from build123d import *

# Parameters (mm, degrees)
SKETCH1_R      = 3.96875
EXTRUDE1_DEPTH = 31.75
CHAMFER1_SIZE  = 0.7874
SKETCH2_W      = 7.62
SKETCH2_H      = 1.27
EXTRUDE2_DEPTH = 6.35


with BuildPart() as part:
    # Sketch1 → Extrude1 (new body)
    with BuildSketch(Plane(origin=(0, 0, 0), x_dir=(0, 0, -1), z_dir=(1, 0, 0))):
        Circle(SKETCH1_R)
    extrude(amount=EXTRUDE1_DEPTH)

    # Chamfer1
    chamfer1_edges = [part.edges().sort_by_distance(p)[0] for p in [
        (0, 0, 3.96875),
        (31.75, 0, 3.96875),
    ]]
    chamfer(chamfer1_edges, length=CHAMFER1_SIZE)

    # Sketch2 → Extrude2 (cut)
    with BuildSketch(Plane(origin=(31.75, 0, 0), x_dir=(0, 0, -1), z_dir=(1, 0, 0))):
        with Locations((0, 3.82905)):
            Rectangle(SKETCH2_W, SKETCH2_H)
    extrude(amount=-EXTRUDE2_DEPTH, mode=Mode.SUBTRACT)


solid = part.part
Read the model definition and answer for the solid it produces. Units are mm, in the model's axes. A direction names the side the tool comes from. Round coordinates to 2 decimals unless told otherwise and drop trailing zeros. Loops run counter-clockwise (first coordinate to the right, second up) from the corner with the lowest first, then second, coordinate; pieces in that order, holes last.
Q1. Which of the six approach directions +Z, -Z, +X, -X, +Y, -Y give full straight-line access (tool end or side, diameter ignored) to faces 1 (the face through (29, 3.194, 0)), 2 (the face through (31.75, 0, 0))?
Q2. Each of these flat-tipped pins is pushed along its axis until it touches: pin 1 (1.5 mm diameter, centred on x = 9, z = 2, fed in from +Y); pin 2 (1.5 mm diameter, centred on x = 25, z = 2.5, fed in from -Y); pin 3 (1 mm diameter, centred on x = 7, y = -2, fed in from +Z). Where does it stop, or does it pass through?
Q3. Consider probe 1 along Y at (x, z) = (2, 1); probe 2 along Z at (x, y) = (18, -3.25); probe 3 along Z at (x, y) = (10, 3). Determine where each line is inside the solid, lowest interval first.
Q4. Section C-C on x = 18 is taken. Write down the section's boundary in (y, z).
Q5. Section B-B on x = 28 is taken. Write down the section's boundary in (y, z).
Output:
1. face 1: +Z, -Z, +X, +Y
1. face 2: +Z, -Z, +X, +Y, -Y
2. pin 1: stops at y = 3.77
2. pin 2: stops at y = -3.56
2. pin 3: stops at z = 3.67
3. probe 1: y = -3.84 to 3.84
3. probe 2: z = -2.28 to 2.28
3. probe 3: z = -2.6 to 2.6
4. outline: circle Ø7.94 at (0, 0)
5. outline: (3.19, -2.36) - (3.19, 2.36) arc R3.97 ccw (long way) to start
